Source: three-view drawing plus pictorial views. Frame: mm from the lowest corner of the part. Give positions to 0.01 mm unless a question says otherwise; leave off trailing zeros. Write each loop counter-clockwise with the first axis right and the second up, starting at its lowest first coordinate (ties: lowest second). Pieces come first, ordered by that corner, then holes. Notation, with made-up numbers: (-4, 12) -> (33, 12) arc R33 ccw to (33, 43) -> close; hole circle Ø1 at (25, -32). An arc over 180 degrees is marked (long way). Answer in a Markdown table with one row per item. Add a question column.
Item 1: Material intervals for probe 1 along Y at (x, z) = (8, 1.75); probe 2 along X at (y, z) = (28.5, 1.8); probe 3 along Y at (x, z) = (29.5, 0.45), sorted ascending. Write a range as from..to.
Item 2: Section query D-D on x = 52. Output: boundary loops of the cut face in (y, z), plus the area to 3 significant figures.
Item 3: Section query C-C on z = 4.35. Output: boundary loops of the cut face in (x, y).
Item 4: Draft query along Y for the marked faces 1, 2 and 3. Return one class per face: +Y half, -Y half, draft (parallel to the pull), parting line (faces both ways), or undercut.
Item 5: Section query A-A on x = 40. Output: boundary loops of the cut face in (y, z), plus the area to 3 significant figures.
Item 6: Section query B-B on y = 30. Output: boundary loops of the cut face in (x, z).
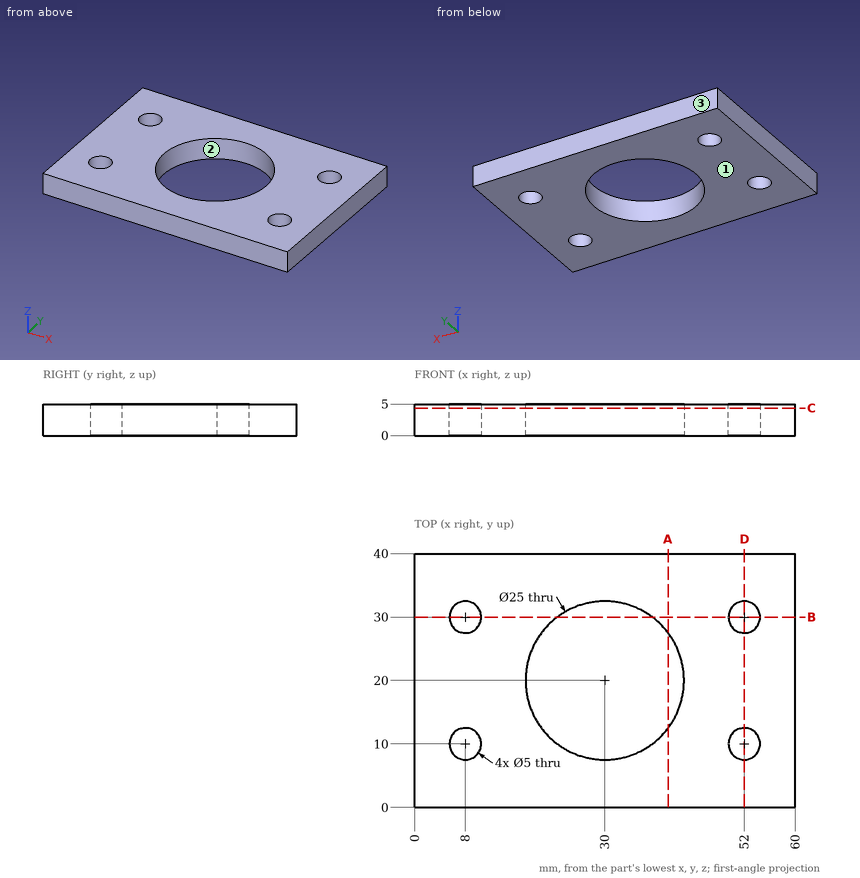
Findings below:
| question | item | result |
|---|---|---|
| 1 | probe 1 | y = 0..7.5, 12.5..27.5, 32.5..40 |
| 1 | probe 2 | x = 0..6, 10..20.83, 39.17..50, 54..60 |
| 1 | probe 3 | y = 0..7.51, 32.49..40 |
| 2 | outline | (0, 0) -> (7.5, 0) -> (7.5, 5) -> (0, 5) -> close; (12.5, 0) -> (27.5, 0) -> (27.5, 5) -> (12.5, 5) -> close; (32.5, 0) -> (40, 0) -> (40, 5) -> (32.5, 5) -> close |
| 2 | area | 150 mm^2 |
| 3 | outline | (0, 0) -> (60, 0) -> (60, 40) -> (0, 40) -> close; hole circle Ø5 at (8, 10); hole circle Ø5 at (8, 30); hole circle Ø25 at (30, 20); hole circle Ø5 at (52, 10); hole circle Ø5 at (52, 30) |
| 4 | face 1 | draft |
| 4 | face 2 | undercut |
| 4 | face 3 | +Y half |
| 5 | outline | (0, 0) -> (12.5, 0) -> (12.5, 5) -> (0, 5) -> close; (27.5, 0) -> (40, 0) -> (40, 5) -> (27.5, 5) -> close |
| 5 | area | 125 mm^2 |
| 6 | outline | (0, 0) -> (5.5, 0) -> (5.5, 5) -> (0, 5) -> close; (10.5, 0) -> (22.5, 0) -> (22.5, 5) -> (10.5, 5) -> close; (37.5, 0) -> (49.5, 0) -> (49.5, 5) -> (37.5, 5) -> close; (54.5, 0) -> (60, 0) -> (60, 5) -> (54.5, 5) -> close |
